from build123d import *

# Parameters (mm, degrees)
SKETCH1_W           = 50.8
SKETCH1_H           = 50.8
SKETCH1_R           = 2.75
SKETCH1_W_2         = 6
SKETCH1_H_2         = 6
BOSS_EXTRUDE1_DEPTH = 7
FILLET1_R           = 2
FILLET2_R           = 4.54


with BuildPart() as part:
    # Sketch1 → Boss-Extrude1 (new body)
    with BuildSketch(Plane(origin=(0, 0, 0), x_dir=(1, 0, 0), z_dir=(0, 1, 0))):
        Rectangle(SKETCH1_W, SKETCH1_H)
        with Locations(Location((0, 0, 0), (0, 0, 270))):
            Circle(SKETCH1_R, mode=Mode.SUBTRACT)
        with Locations((-19.4, 19.4)):
            Rectangle(SKETCH1_W_2, SKETCH1_H_2, mode=Mode.SUBTRACT)
        with Locations((19.4, 19.4)):
            Rectangle(SKETCH1_W_2, SKETCH1_H_2, mode=Mode.SUBTRACT)
        with Locations((-19.4, -19.4)):
            Rectangle(SKETCH1_W_2, SKETCH1_H_2, mode=Mode.SUBTRACT)
        with Locations((19.4, -19.4)):
            Rectangle(SKETCH1_W_2, SKETCH1_H_2, mode=Mode.SUBTRACT)
    extrude(amount=BOSS_EXTRUDE1_DEPTH)

    # Fillet1
    fillet1_edges = [part.edges().sort_by_distance(p)[0] for p in [
        (0, 0, 25.4),
        (-25.4, 0, 0),
        (0, 0, -25.4),
        (25.4, 0, 0),
    ]]
    fillet(fillet1_edges, radius=FILLET1_R)

    # Fillet2
    # the kernel refuses this fillet: 4.54 mm, written as the material it takes off along each edge
    with BuildSketch(Plane(origin=(20.86, 0, -20.86), x_dir=(0, 0, -1), z_dir=(-1, 0, 0))) as fillet2_piece_1:
        with BuildLine():
            CenterArc((2.54, -2), 2, 0, 90)
            Line((4.54, -2), (4.54, 0))
            Line((4.54, 0), (2.54, 0))
        make_face()
    revolve(axis=Axis((20.86, 0, -20.86), (0, -1, 0)), revolution_arc=90, mode=Mode.SUBTRACT)
    with BuildSketch(Plane(origin=(20.86, 0, 20.86), x_dir=(1, 0, 0), z_dir=(0, 0, -1))) as fillet2_piece_2:
        with BuildLine():
            CenterArc((2.54, -2), 2, 0, 90)
            Line((4.54, -2), (4.54, 0))
            Line((4.54, 0), (2.54, 0))
        make_face()
    revolve(axis=Axis((20.86, 0, 20.86), (0, -1, 0)), revolution_arc=90, mode=Mode.SUBTRACT)
    with BuildSketch(Plane(origin=(-20.86, 0, -20.86), x_dir=(-1, 0, 0), z_dir=(0, 0, 1))) as fillet2_piece_3:
        with BuildLine():
            CenterArc((2.54, -2), 2, 0, 90)
            Line((4.54, -2), (4.54, 0))
            Line((4.54, 0), (2.54, 0))
        make_face()
    revolve(axis=Axis((-20.86, 0, -20.86), (0, -1, 0)), revolution_arc=90, mode=Mode.SUBTRACT)
    with BuildSketch(Plane(origin=(-20.86, 0, 20.86), x_dir=(0, 0, 1), z_dir=(1, 0, 0))) as fillet2_piece_4:
        with BuildLine():
            CenterArc((2.54, -2), 2, 0, 90)
            Line((4.54, -2), (4.54, 0))
            Line((4.54, 0), (2.54, 0))
        make_face()
    revolve(axis=Axis((-20.86, 0, 20.86), (0, -1, 0)), revolution_arc=90, mode=Mode.SUBTRACT)
    with BuildSketch(Plane(origin=(25.4, 0, 25.4), x_dir=(0, 0, -1), z_dir=(0, 1, 0)), Plane(origin=(25.4, 0, -25.4), x_dir=(-1, 0, 0), z_dir=(0, 1, 0))) as fillet2_piece_5:
        with BuildLine():
            CenterArc((FILLET2_R, FILLET2_R), FILLET2_R, 180, 90)
            Line((0, FILLET2_R), (0, 0))
            Line((0, 0), (FILLET2_R, 0))
        make_face()
    extrude(amount=18.35, mode=Mode.SUBTRACT)
    with BuildSketch(Plane(origin=(-25.4, 0, 25.4), x_dir=(0, 0, -1), z_dir=(0, 1, 0)), Plane(origin=(-25.4, 0, -25.4), x_dir=(1, 0, 0), z_dir=(0, 1, 0))) as fillet2_piece_6:
        with BuildLine():
            CenterArc((FILLET2_R, -FILLET2_R), FILLET2_R, 90, 90)
            Line((0, -FILLET2_R), (0, 0))
            Line((0, 0), (FILLET2_R, 0))
        make_face()
    extrude(amount=18.35, mode=Mode.SUBTRACT)


solid = part.part
Read the model definition and answer for the solid it produces. Units are mm, in the model's axes. A direction names the side the tool comes from. Coordinates: 2 decimals unless noted, no trailing zeros. Order: outer loops, then holes, each group sorted by start corner. A loop starts at its lowest first (then second) coordinate and runs counter-clockwise, first axis right, second up. Notation, with made-up numbers: (30.25, -34.5) -> (77.25, -34.5) arc R23 cw to (77.25, 3.5) -> close; hole circle Ø4 at (70, 30). An arc over 180 degrees is marked (long way). Answer as a JSON object with one key per item and string values.
1) A cutting plane is placed at D-D, the plane x = -17.5. Determine the outline of the cut face in (y, z), plus the area to 3 significant figures.
Model answer:
{"outline": "(0, -23.4) arc R2 ccw to (2, -25.4) -> (7, -25.4) -> (7, -22.4) -> (0, -22.4) -> close; (0, -16.4) -> (7, -16.4) -> (7, 16.4) -> (0, 16.4) -> close; (0, 22.4) -> (7, 22.4) -> (7, 25.4) -> (2, 25.4) arc R2 ccw to (0, 23.4) -> close", "area": "270 mm²"}
2) A tool of negligible diameter and unlimited length cuts with its end or side. For faces 5 (the face through (19, 3, 16.4)), 6 (the face through (0, 4, -25.4)), from which of +Z, -Z, +X, -X, +Y, -Y can it reach the whole face along a straight path? Write none if from no direction.
Model answer:
{"face 5": "+Y, -Y", "face 6": "-Z, +X, -X, +Y, -Y"}
3) A cutting plane is placed at B-B, the plane y = 3.25. Determine the outline of the cut face in (x, z), plus the area to 3 significant figures.
Model answer:
{"outline": "(-25.4, -20.86) arc R4.54 ccw to (-20.86, -25.4) -> (20.86, -25.4) arc R4.54 ccw to (25.4, -20.86) -> (25.4, 20.86) arc R4.54 ccw to (20.86, 25.4) -> (-20.86, 25.4) arc R4.54 ccw to (-25.4, 20.86) -> close; hole (-22.4, -22.4) -> (-16.4, -22.4) -> (-16.4, -16.4) -> (-22.4, -16.4) -> close; hole (-22.4, 16.4) -> (-16.4, 16.4) -> (-16.4, 22.4) -> (-22.4, 22.4) -> close; hole circle Ø5.5 at (0, 0); hole (16.4, -22.4) -> (22.4, -22.4) -> (22.4, -16.4) -> (16.4, -16.4) -> close; hole (16.4, 16.4) -> (22.4, 16.4) -> (22.4, 22.4) -> (16.4, 22.4) -> close", "area": "2,400 mm²"}
4) The mould has two halves that part along Z. Classify faces 1 (the face through (0.29, 0.6, -24.83)), 2 (the face through (-24.11, 4.46, 24.03)), 3 (the face through (-25.4, 4, 0)), 4 (the face through (-16.4, 3, 19)): released by +Z, released by -Z, zero draft, split by the parting line, or undercut.
Model answer:
{"face 1": "released by -Z", "face 2": "released by +Z", "face 3": "zero draft", "face 4": "undercut"}
5) Consider line 1 along X through (y, z) = (3.5, -19); line 2 along X through (y, z) = (4.75, 0). Determine where each line is inside the solid, lowest interval first. Write a range as from..to.
Model answer:
{"line 1": "x = -25.4..-22.4, -16.4..16.4, 22.4..25.4", "line 2": "x = -25.4..-2.75, 2.75..25.4"}
6) A cutting plane is placed at C-C, the plane x = 0. Determine the outline of the cut face in (y, z), plus the area to 3 significant figures.
Model answer:
{"outline": "(0, -23.4) arc R2 ccw to (2, -25.4) -> (7, -25.4) -> (7, -2.75) -> (0, -2.75) -> close; (0, 2.75) -> (7, 2.75) -> (7, 25.4) -> (2, 25.4) arc R2 ccw to (0, 23.4) -> close", "area": "315 mm²"}
7) A cutting plane is placed at A-A, the plane z = 0. Determine the outline of the cut face in (x, y).
Model answer:
{"outline": "(-25.4, 2) arc R2 ccw to (-23.4, 0) -> (-2.75, 0) -> (-2.75, 7) -> (-25.4, 7) -> close; (2.75, 0) -> (23.4, 0) arc R2 ccw to (25.4, 2) -> (25.4, 7) -> (2.75, 7) -> close"}
